from build123d import *

# Parameters (mm, degrees)
F0_W     = 762
F0_H     = 381
F1_DEPTH = 431.8
F2_DEPTH = 25.4
F3_T     = -6.35


with BuildPart() as f1:
    # F0 (on Top) → F1 (new body)
    with BuildSketch(Plane.XY):
        with Locations((-381, -190.5)):
            Rectangle(F0_W, F0_H)
    extrude(amount=F1_DEPTH)

    # F2 (add): a face of the model
    f2_faces = [f1.faces().sort_by_distance(p)[0] for p in [
        (-381, -190.5, 431.8),
    ]]
    extrude(f2_faces, amount=F2_DEPTH)

    # F3
    f3_openings = [f1.faces().sort_by_distance(p)[0] for p in [
        (-381, -190.5, 457.2),
    ]]
    offset(amount=F3_T, openings=f3_openings)


solid = f1.part
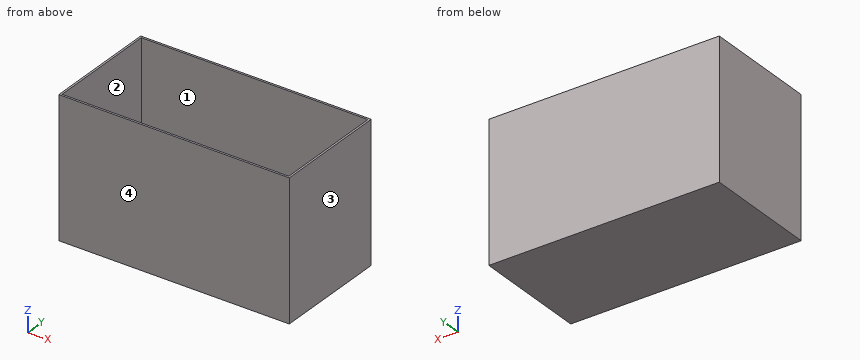
Part model, mm, in its own coordinate system. Face numbers are marked on the shaded views. Round coordinates to 2 decimals unless told otherwise and drop trailing zeros. Write each loop counter-clockwise with the first axis right and the second up, starting at its lowest first coordinate (ties: lowest second). Pieces come first, ordered by that corner, then holes. Notation, with made-up numbers: M 12.25,7 L 38.25,7 A11 ccw 38.25,22 Z; hole C -39.75,4.5 d2. An arc over 180 degrees is marked long. Return JSON: item names as keys, results as strings. Group by question number.
(1) Pin check, flat tip, straight feed: pin 1 Ø12 at (x, y) = (-657.5, -117) entering from +Z. Stop position of the tip, or through.
(2) Saw through at A-A on z = 85.5. Write the cut outline in (x, y), then the cut area to 3 significant figures.
(3) Drill centre lines: probe 1 along X at (y, z) = (-232.5, 324.5); probe 2 along Y at (x, z) = (-726, 273.5); probe 3 along Z at (x, y) = (-185, -279.5). Where is each one in solid material? Low to high.
(4) Two-plate mould, pull along Y, no slides. Class the marked faces 1, 2, 3 and 4: +Y half, -Y half, draft (parallel to the pull), parting line (faces both ways), or undercut.
(5) Saw through at B-B on x = -587.5. Write the cut outline in (y, z), then the cut area to 3 significant figures.
(6) Saw through at C-C on y = -164. Write the cut outline in (x, z).
Returned:
{
 "1": {"pin 1": "z = 6.35"},
 "2": {"outline": "M -762,-381 L 0,-381 L 0,0 L -762,0 Z; hole M -755.65,-374.65 L -6.35,-374.65 L -6.35,-6.35 L -755.65,-6.35 Z", "area": "14,400 mm²"},
 "3": {"probe 1": "-762 to -755.65, -6.35 to 0", "probe 2": "-381 to -374.65, -6.35 to 0", "probe 3": "0 to 6.35"},
 "4": {"face 1": "undercut", "face 2": "undercut", "face 3": "draft", "face 4": "-Y half"},
 "5": {"outline": "M -381,0 L 0,0 L 0,457.2 L -6.35,457.2 L -6.35,6.35 L -374.65,6.35 L -374.65,457.2 L -381,457.2 Z", "area": "8,150 mm²"},
 "6": {"outline": "M -762,0 L 0,0 L 0,457.2 L -6.35,457.2 L -6.35,6.35 L -755.65,6.35 L -755.65,457.2 L -762,457.2 Z"}
}
